Autodesk Inventor part; units mm, degrees
ref_plane "YZ Plane" through (0, 0, 0) normal (1, 0, 0) x (0, 1, 0)
ref_plane "XZ Plane" through (0, 0, 0) normal (0, 1, 0) x (-1, 0, 0)
ref_plane "XY Plane" through (0, 0, 0) normal (0, 0, 1) x (1, 0, 0)
sketch "Sketch1" plane through (0, 0, 0) normal (0, 1, 0) x (-1, 0, 0)
  line L0 (0, 0) -> (113.5, 0)
  line L1 (113.5, 0) -> (113.5, -111)
  line L2 (113.5, -111) -> (0, -111)
  line L3 (0, -111) -> (0, 0)
  dimension "d0" = 113.5
  dimension "d1" = 111
extrude "Extrusion1" add sketch "Sketch1" along normal blind 35
sketch "Sketch2" plane through (0, 0, 0) normal (1, 0, 0) x (0, 0, -1)
  line L0 (0, 0) -> (0, 4.5)
  line L1 (0, 4.5) -> (8, 4.5)
  line L2 (8, 4.5) -> (103, 4.5)
  line L3 (103, 4.5) -> (103, 30.5)
  line L4 (103, 30.5) -> (8, 30.5)
  line L5 (8, 30.5) -> (8, 4.5)
  dimension "d4" = 4.5
  dimension "d5" = 8
  dimension "d6" = 95
  dimension "d7" = 26
extrude "Extrusion2" cut sketch "Sketch2" against normal blind 112
sketch "Sketch3" plane through (-112, 0, 0) normal (1, 0, 0) x (0, 0, -1)
  line L0 (8, 4.5) -> (8, 30.5)
  line L1 (8, 4.5) -> (44, 4.5)
  line L2 (103, 4.5) -> (8, 4.5)
  line L3 (8, 4.5) -> (8, 14.5)
  line L4 (8, 14.5) -> (44, 14.5)
  line L5 (44, 14.5) -> (44, 4.5)
  point P0 (0, 0)
  dimension "d10" = 36
  dimension "d11" = 10
extrude "Extrusion3" add sketch "Sketch3" along normal blind 20
sketch "Sketch4" plane through (0, 0, 0) normal (1, 0, 0) x (0, 0, -1)
  line L0 (0, 0) -> (0, 7)
  line L1 (0, 7) -> (5, 7)
  line L2 (5, 7) -> (5, 14)
  line L3 (5, 14) -> (8, 14)
  line L4 (8, 4.5) -> (8, 30.5)
  line L5 (5, 7) -> (8, 7)
  line L6 (8, 14) -> (8, 7)
  line L7 (111, 0) -> (111, 6.5)
  line L8 (111, 6.5) -> (106, 6.5)
  line L9 (106, 6.5) -> (106, 11.5)
  line L10 (103, 30.5) -> (103, 4.5)
  line L11 (106, 6.5) -> (103, 6.5)
  line L12 (106, 11.5) -> (103, 11.5)
  line L13 (103, 6.5) -> (103, 11.5)
  line L14 (103, 6.5) -> (103, 9)
  line L15 (103, 30.5) -> (103, 4.5)
  line L16 (103, 9) -> (106, 9)
  line L17 (8, 7) -> (8, 10.5)
  line L18 (5, 10.5) -> (8, 10.5)
  dimension "d14" = 7
  dimension "d15" = 5
  dimension "d16" = 7
  dimension "d17" = 6.5
  dimension "d18" = 5
  dimension "d19" = 5
extrude "Extrusion4" cut sketch "Sketch4" against normal blind 95 contours L2 L3 L4 L18 | L16 L10 L12 L9
properties part number "Plastic_Housing" material "Polyethylene, High Density"
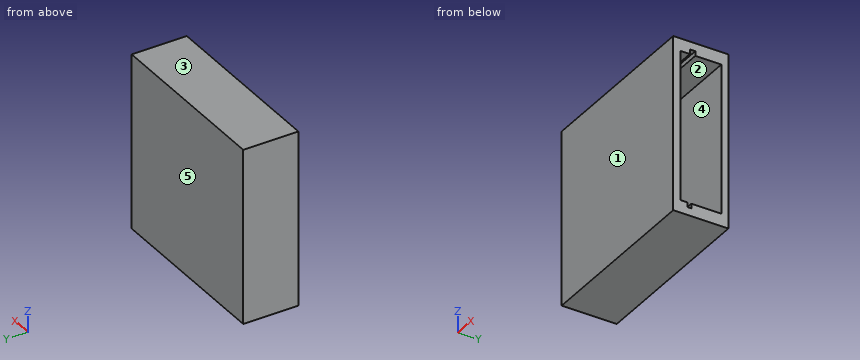
The listing builds one solid part. Answer for the finished solid, in the listing's coordinates (mm). Face numbers are marked on the shaded views. A direction names the side the tool comes from. Give positions to 0.01 mm unless a question says otherwise; leave off trailing zeros. Order: outer loops, then holes, each group sorted by start corner. A loop starts at its lowest first (then second) coordinate and runs counter-clockwise, first axis right, second up. Notation, with made-up numbers: (88.5, -32) - (109.5, -32) arc R20 ccw to (109.5, 2) - close; hole circle Ø6 at (63, 88.5). An arc over 180 degrees is marked (long way). Answer in a Markdown table with one row per item. Add a question column.
Q1. The part is cut by section C-C (y = 17). Determine the outline of the cut face in (x, z), then the cut area to 3 significant figures.
Q2. The part is cut by section D-D (z = -23). Determine the outline of the cut face in (x, y), then the cut area to 3 significant figures.
Q3. Given P1, Ø8, axis at x = -39, y = 18, coming from the +Z side; P2, Ø1, axis at y = 12, z = -14.5, coming from the +X side; P3, Ø1.5, axis at y = 12, z = -6.5, coming from the +X side, each flat-ended and moving along its own axis, determine where each tip first touches the part or whether it passes through.
Q4. The part is cut by section A-A (x = -57). Determine the outline of the cut face in (y, z).
Q5. The part is cut by section B-B (z = -69.5). Determine the outline of the cut face in (x, y).
Q6. Which of the six approach directions +Z, -Z, +X, -X, +Y, -Y give full straight-line access (tool end or side, diameter ignored) to the marked faces 4 and 5?
Q7. For a pull along Y with two mould halves and no side action, classify the marked faces 1, 2 and 3 as released by +Y, released by -Y, zero draft, split by the parting line, or undercut.
Q8. Find the intervals of material crossed by line 1 along Y through (x, z) = (-32.5, -27.5); line 2 along Z through (x, y) = (-8, 18); line 3 along Y through (x, z) = (-95.5, -30), in increasing order. Write a range as [from, to].
Determined:
| question | item | result |
|---|---|---|
| 1 | outline | (-113.5, -111) - (0, -111) - (0, -103) - (-112, -103) - (-112, -8) - (0, -8) - (0, 0) - (-113.5, 0) - close |
| 1 | area | 1,960 mm² |
| 2 | outline | (-113.5, 0) - (0, 0) - (0, 4.5) - (-92, 4.5) - (-92, 14.5) - (-112, 14.5) - (-112, 30.5) - (0, 30.5) - (0, 35) - (-113.5, 35) - close |
| 2 | area | 1,260 mm² |
| 3 | P1 | stops at z = 0 |
| 3 | P2 | stops at x = -92 |
| 3 | P3 | stops at x = -95 |
| 4 | outline | (0, -111) - (35, -111) - (35, 0) - (0, 0) - close; hole (4.5, -103) - (9, -103) - (9, -106) - (11.5, -106) - (11.5, -103) - (30.5, -103) - (30.5, -8) - (14, -8) - (14, -5) - (10.5, -5) - (10.5, -8) - (4.5, -8) - close |
| 5 | outline | (-113.5, 0) - (0, 0) - (0, 4.5) - (-112, 4.5) - (-112, 30.5) - (0, 30.5) - (0, 35) - (-113.5, 35) - close |
| 6 | face 4 | +X |
| 6 | face 5 | +Z, -Z, +X, -X, +Y |
| 7 | face 1 | released by -Y |
| 7 | face 2 | undercut |
| 7 | face 3 | zero draft |
| 8 | line 1 | y = [0, 4.5], [30.5, 35] |
| 8 | line 2 | z = [-111, -103], [-8, 0] |
| 8 | line 3 | y = [0, 14.5], [30.5, 35] |
